For this review, use the dimensioned drawing (mm, ordinates from the lowest corner) and the shaded views. Coordinates: 2 decimals unless noted, no trailing zeros. Order: outer loops, then holes, each group sorted by start corner. A loop starts at its lowest first (then second) coordinate and runs counter-clockwise, first axis right, second up. Notation, with made-up numbers: M 46.25,81 L 90.25,81 A19 cw 90.25,90 Z; hole C 35.25,56 d6. An arc over 180 degrees is marked long. One line per item, written item: value.
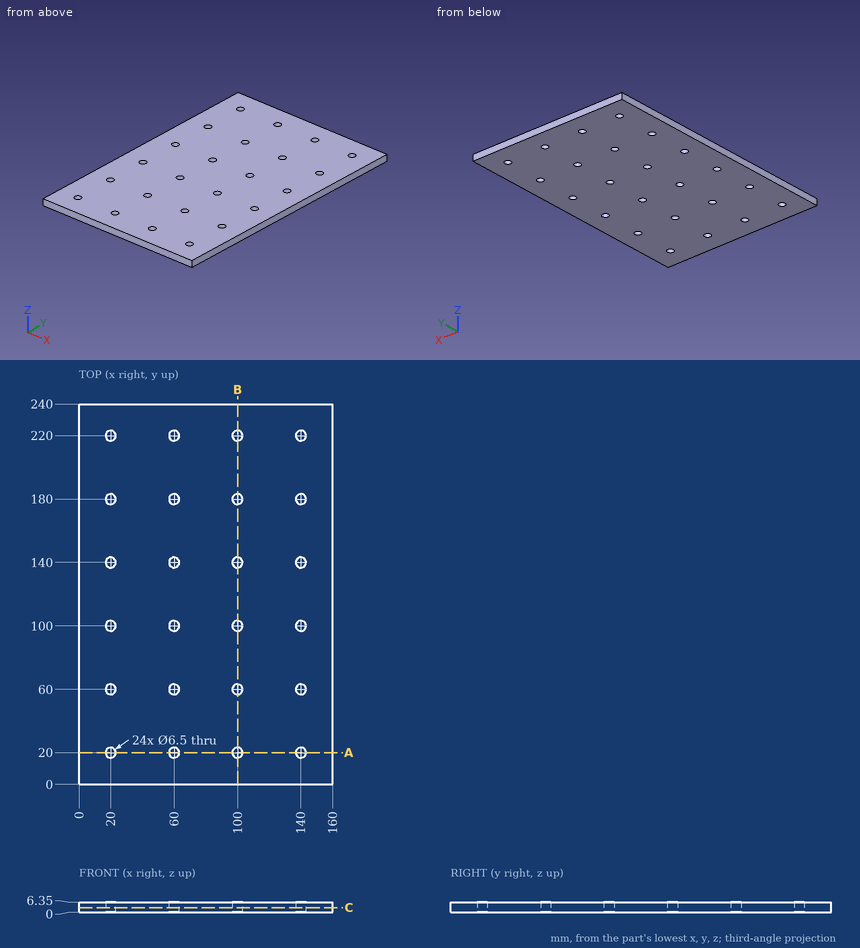
(1) For L1, parallel to X at y = 180, z = 2.5, list the stretches that pass through material, from the lowest coordinate up.
Geometry results:
L1: x = 0 to 16.75, 23.25 to 56.75, 63.25 to 96.75, 103.25 to 136.75, 143.25 to 160
(2) Insertion check: pin 1 Ø6 at (x, y) = (60, 60) entering from -Z; pin 2 Ø10.5 at (x, y) = (140, 180) entering from -Z. Each pin has a flat end and moves straight along its axis. Give the tip position at first contact, or say it passes through.
Geometry results:
pin 1: passes through
pin 2: stops at z = 0
(3) We need section A-A, the plane y = 20. State the section outline as (x, z) points.
Geometry results:
outline: M 0,0 L 16.75,0 L 16.75,6.35 L 0,6.35 Z; M 23.25,0 L 56.75,0 L 56.75,6.35 L 23.25,6.35 Z; M 63.25,0 L 96.75,0 L 96.75,6.35 L 63.25,6.35 Z; M 103.25,0 L 136.75,0 L 136.75,6.35 L 103.25,6.35 Z; M 143.25,0 L 160,0 L 160,6.35 L 143.25,6.35 Z
(4) We need section C-C, the plane z = 3. Count the separate pieces of the cut face and the enclosed holes in it, plus the area to 3 significant figures.
Geometry results:
separate pieces: 1
enclosed holes: 24
area: 37,600 mm2
(5) We need section B-B, the plane x = 100. State the section outline as (y, z) points, plus the area to 3 significant figures.
Geometry results:
outline: M 0,0 L 16.75,0 L 16.75,6.35 L 0,6.35 Z; M 23.25,0 L 56.75,0 L 56.75,6.35 L 23.25,6.35 Z; M 63.25,0 L 96.75,0 L 96.75,6.35 L 63.25,6.35 Z; M 103.25,0 L 136.75,0 L 136.75,6.35 L 103.25,6.35 Z; M 143.25,0 L 176.75,0 L 176.75,6.35 L 143.25,6.35 Z; M 183.25,0 L 216.75,0 L 216.75,6.35 L 183.25,6.35 Z; M 223.25,0 L 240,0 L 240,6.35 L 223.25,6.35 Z
area: 1,280 mm2
